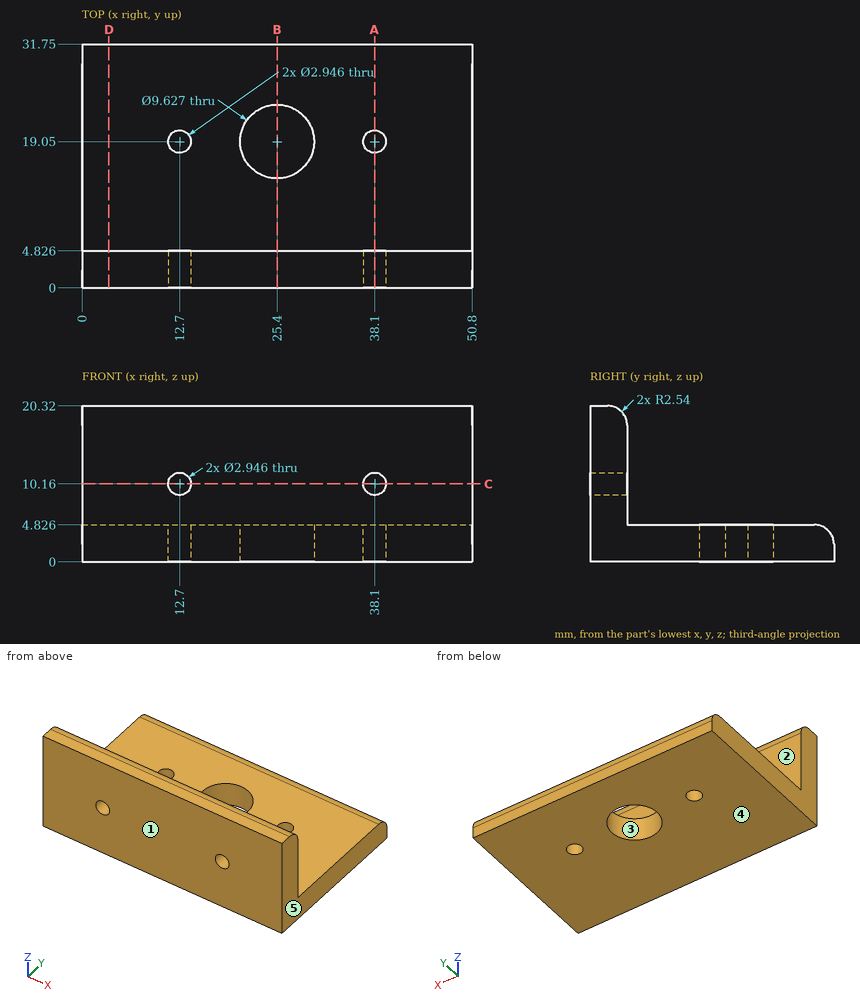
For this review, use the dimensioned drawing (mm, ordinates from the lowest corner) and the shaded views. A direction names the side the tool comes from. Give positions to 0.01 mm unless a question says otherwise; leave off trailing zeros. Order: outer loops, then holes, each group sorted by start corner. A loop starts at its lowest first (then second) coordinate and runs counter-clockwise, first axis right, second up. Notation, with made-up numbers: (16.5, 68.5) - (35.5, 68.5) arc R21 cw to (35.5, 103.5) - close; hole circle Ø3 at (30, -7). An arc over 180 degrees is marked (long way). Use a Markdown table: item, result. Add a question column.
(1) Add section B-B on x = 25.4. Give the boundary of the cut face in (y, z).
(2) Add section A-A on x = 38.1. Give the boundary of the cut face in (y, z), then the cut area to 3 significant figures.
(3) Add section C-C on z = 10.16. Give the boundary of the cut face in (x, y), then the cut area to 3 significant figures.
(4) Machinability: for the marked faces 1 and 2, which of the approach directions +Z, -Z, +X, -X, +Y, -Y give a long, thin tool a straight path to every point of the face, cutting with its end or side? Answer none if there is none.
(5) Add section D-D on x = 3.5. Give the boundary of the cut face in (y, z).
(6) Mouldability with a two-part tool opening along X and no side actions: class the marked faces 3, 4 and 5 as +X half, -X half, draft (parallel to the pull), parting line (faces both ways), or undercut.
(7) Wall thickness on probe 1 along X at (y, z) = (3.8, 10.16); probe 2 along Y at (x, z) = (38.1, 1.85); probe 3 along Y at (x, z) = (12.5, 7.5): over which ranges is each line inside the solid? List them lowest first. Write a range as [from, to].
(8) Clearance check with flat-ended pins moving along their axes: P1, Ø6, axis at x = 23.5, y = 8, coming from the +Z side; P2, Ø2, axis at x = 26, y = 12, coming from the -Z side; P3, Ø6.5, axis at x = 22.5, z = 10.5, coming from the +Y side; P4, Ø5, axis at x = 43.5, z = 5.5, coming from the +Y side. State where each tip first meets the part, or that it passes through.
Report:
| question | item | result |
|---|---|---|
| 1 | outline | (0, 0) - (14.24, 0) - (14.24, 4.83) - (4.83, 4.83) - (4.83, 17.78) arc R2.54 ccw to (2.29, 20.32) - (0, 20.32) - close; (23.86, 0) - (31.75, 0) - (31.75, 2.29) arc R2.54 ccw to (29.21, 4.83) - (23.86, 4.83) - close |
| 2 | outline | (0, 0) - (17.58, 0) - (17.58, 4.83) - (4.83, 4.83) - (4.83, 8.69) - (0, 8.69) - close; (0, 11.63) - (4.83, 11.63) - (4.83, 17.78) arc R2.54 ccw to (2.29, 20.32) - (0, 20.32) - close; (20.52, 0) - (31.75, 0) - (31.75, 2.29) arc R2.54 ccw to (29.21, 4.83) - (20.52, 4.83) - close |
| 2 | area | 197 mm² |
| 3 | outline | (0, 0) - (11.23, 0) - (11.23, 4.83) - (0, 4.83) - close; (14.17, 0) - (36.63, 0) - (36.63, 4.83) - (14.17, 4.83) - close; (39.57, 0) - (50.8, 0) - (50.8, 4.83) - (39.57, 4.83) - close |
| 3 | area | 217 mm² |
| 4 | face 1 | +Z, -Z, +X, -X, -Y |
| 4 | face 2 | +Z, +X, -X, +Y |
| 5 | outline | (0, 0) - (31.75, 0) - (31.75, 2.29) arc R2.54 ccw to (29.21, 4.83) - (4.83, 4.83) - (4.83, 17.78) arc R2.54 ccw to (2.29, 20.32) - (0, 20.32) - close |
| 6 | face 3 | undercut |
| 6 | face 4 | draft |
| 6 | face 5 | +X half |
| 7 | probe 1 | x = [0, 11.23], [14.17, 36.63], [39.57, 50.8] |
| 7 | probe 2 | y = [0, 17.58], [20.52, 31.75] |
| 7 | probe 3 | y = [0, 4.83] |
| 8 | P1 | stops at z = 4.83 |
| 8 | P2 | stops at z = 0 |
| 8 | P3 | stops at y = 4.83 |
| 8 | P4 | stops at y = 31.65 |
